The listing builds one solid part. Answer for the finished solid, in the listing's coordinates (mm). A direction names the side the tool comes from. Give positions to 0.01 mm unless a question says otherwise; leave off trailing zeros. Order: outer loops, then holes, each group sorted by start corner. A loop starts at its lowest first (then second) coordinate and runs counter-clockwise, first axis right, second up. Notation, with made-up numbers: (-29.75, 46.5) - (15.25, 46.5) arc R27 cw to (15.25, 79.5) - close; hole circle Ø8 at (12.5, 21.25). An arc over 180 degrees is marked (long way). Use a Markdown table: item, result. Add a question column.
1) For faces 5 (the face through (95.39, 4.84, -4.97)), 6 (the face through (51.16, 18.58, -2.46)), 7 (the face through (95.382, -27.918, -4.93)), determine the directions among +Z, -Z, +X, -X, +Y, -Y from which every point of the face is accessible in a straight line to the end or side of a thin tool.
2) Flat-ended cylindrical pins translate along their axes: pin 1 (5 mm diameter, centred on x = 84.12, y = 37.28, fed in from +Z); pin 2 (2 mm diameter, centred on y = 32.5, z = -8, fed in from +X); pin 3 (5 mm diameter, centred on y = 26.5, z = -4, fed in from +X). Find the tip coordinate at first contact, or state that the pin passes through.
3) Straight lines are drawn through the part: line 1 (X direction, y = 35.5, z = -5.5); line 2 (X direction, y = -13.5, z = -2.5); line 3 (Y direction, x = 89, z = -4.25). For each, find the intervals that lie inside material, in ascending order.
4) Find section A-A, the plane x = 92.5. Determine the outline of the cut face in (y, z).
5) Find section B-B, the plane y = -10. State how many separate pieces and enclosed holes the cut face has, plus the area to 3 significant figures.
6) The mould has two halves that part along X. Classify faces 1 (the face through (107.529, 6.016, -4.93)), 2 (the face through (73.77, 3.88, -5.03)), 3 (the face through (107.2, 5.15, -4.97)), 4 (the face through (52.91, 4.84, -4.93)): released by +X, released by -X, zero draft, split by the parting line, or undercut.
from build123d import *

# Parameters (mm, degrees)
BOSS_EXTRUDE1_DEPTH = 10
SKETCH2_R           = 2
CUT_EXTRUDE1_DEPTH  = 139.371645796
CUT_EXTRUDE2_START  = -4
SKETCH2_3_R         = 2
CUT_EXTRUDE2_DEPTH  = 135.371645796
SKETCH3_R           = 2
CUT_EXTRUDE3_DEPTH  = 35
SKETCH4_R           = 2
CUT_EXTRUDE4_DEPTH  = 10
SKETCH4_3_R         = 2
CUT_EXTRUDE5_DEPTH  = 5


with BuildPart() as part:
    # Sketch1 → Boss-Extrude1 (new body)
    with BuildSketch(Plane.XY):
        Polygon((127.346442995, -36.483176399), (87.147938799, 49.722794044), (41.832549447, 28.591880957), (64.300112266, -19.589962995), align=None)
    extrude(amount=-BOSS_EXTRUDE1_DEPTH)

    # Sketch2 → Cut-Extrude1 (cut, through all)
    with BuildSketch(Plane(origin=(-3.479773272, 7.462397864, 0), x_dir=(0.9063077870366519, 0.4226182617406953, 0), z_dir=(-0.42261826174069533, 0.906307787036652, 0))):
        with Locations(Location((64.996616346, 5, 0), (0, 0, 180))):
            Circle(SKETCH2_R)
        with Locations(Location((84.996616346, 5, 0), (0, 0, 180))):
            Circle(SKETCH2_R)
    extrude(amount=-CUT_EXTRUDE1_DEPTH, mode=Mode.SUBTRACT)

    # Sketch2<3> → Cut-Extrude2 (cut, through all)
    # profile 1 of 2: a face of its own
    with BuildSketch(Plane(origin=(-3.479773272, 7.462397864, 0), x_dir=(0.9063077870366519, 0.4226182617406953, 0), z_dir=(-0.42261826174069533, 0.906307787036652, 0)).offset(CUT_EXTRUDE2_START)):
        Polygon((84.996616346, 0.958548116), (88.496616346, 2.979274058), (88.496616346, 7.020725942), (84.996616346, 9.041451884), (81.496616346, 7.020725942), (81.496616346, 2.979274058), align=None)
        with Locations(Location((84.996616346, 5, 0), (0, 0, 180))):
            Circle(SKETCH2_3_R, mode=Mode.SUBTRACT)
    # profile 2 of 2: a face of its own
    with BuildSketch(Plane(origin=(-3.479773272, 7.462397864, 0), x_dir=(0.9063077870366519, 0.4226182617406953, 0), z_dir=(-0.42261826174069533, 0.906307787036652, 0)).offset(CUT_EXTRUDE2_START)):
        Polygon((68.496616346, 2.979274058), (64.996616346, 0.958548116), (61.496616346, 2.979274058), (61.496616346, 7.020725942), (64.996616346, 9.041451884), (68.496616346, 7.020725942), align=None)
        with Locations(Location((64.996616346, 5, 0), (0, 0, 180))):
            Circle(SKETCH2_3_R, mode=Mode.SUBTRACT)
    extrude(amount=-CUT_EXTRUDE2_DEPTH, mode=Mode.SUBTRACT)

    # Sketch3 → Cut-Extrude3 (cut)
    with BuildSketch(Plane(origin=(-0.59019996, -2.202656237, 0), x_dir=(0.9659258262890685, -0.2588190451025201, 0), z_dir=(-0.2588190451025201, -0.9659258262890685, 0))):
        with Locations((82.809116935, -5)):
            Circle(SKETCH3_R)
        with Locations((102.893564909, -5)):
            Circle(SKETCH3_R)
    extrude(amount=-CUT_EXTRUDE3_DEPTH, mode=Mode.SUBTRACT)

    # Sketch4 → Cut-Extrude4 (cut)
    with BuildSketch(Plane.XY):
        with Locations((84.12365912, 37.27877008)):
            Circle(SKETCH4_R)
        with Locations((51.496578787, 22.064512657)):
            Circle(SKETCH4_R)
    extrude(amount=-CUT_EXTRUDE4_DEPTH, mode=Mode.SUBTRACT)

    # Sketch4<3> → Cut-Extrude5 (cut)
    # profile 1 of 2: a face of its own
    with BuildSketch(Plane.XY):
        Polygon((88.14973206, 36.926534339), (86.44174069, 40.589333653), (82.41566775, 40.941569394), (80.09758618, 37.631005821), (81.805577551, 33.968206507), (85.83165049, 33.615970766), align=None)
        with Locations((84.12365912, 37.27877008)):
            Circle(SKETCH4_3_R, mode=Mode.SUBTRACT)
    # profile 2 of 2: a face of its own
    with BuildSketch(Plane.XY):
        Polygon((55.522651726, 21.712276917), (53.814660356, 25.37507623), (49.788587416, 25.727311971), (47.470505847, 22.416748398), (49.178497217, 18.753949084), (53.204570157, 18.401713344), align=None)
        with Locations((51.496578787, 22.064512657)):
            Circle(SKETCH4_3_R, mode=Mode.SUBTRACT)
    extrude(amount=-CUT_EXTRUDE5_DEPTH, mode=Mode.SUBTRACT)


solid = part.part
The answers:
| question | item | result |
|---|---|---|
| 1 | face 5 | none |
| 1 | face 6 | +Z |
| 1 | face 7 | +Z, -Z, -X, -Y |
| 2 | pin 1 | z = -5 |
| 2 | pin 2 | x = 95.65 |
| 2 | pin 3 | x = 99.14 |
| 3 | line 1 | 57.3 to 73.37, 81.09 to 83.21, 85.04 to 93.78 |
| 3 | line 2 | 61.46 to 75.07, 80.96 to 97.13, 103.02 to 116.63 |
| 3 | line 3 | -26.21 to 1.98, 18.54 to 45.75 |
| 4 | outline | (-27.15, -10) - (38.25, -10) - (38.25, 0) - (-27.15, 0) - close; hole (-5.53, -7.02) - (2.75, -9.04) - (11.03, -7.02) - (11.03, -2.98) - (2.75, -0.96) - (-5.53, -2.98) - close |
| 5 | separate pieces | 1 |
| 5 | enclosed holes | 3 |
| 5 | area | 433 mm2 |
| 6 | face 1 | released by +X |
| 6 | face 2 | undercut |
| 6 | face 3 | undercut |
| 6 | face 4 | released by -X |
